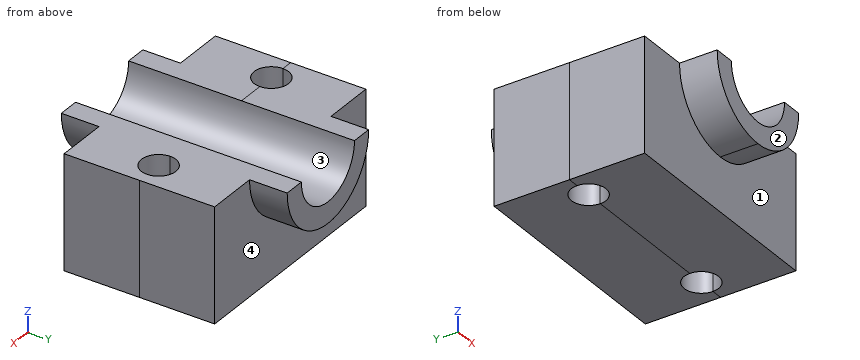
from build123d import *
from build123d import SkipClean  # not in build123d's __all__

# Parameters (mm, degrees)
F1_DEPTH = 25.4
F2_DEPTH = 12.7
F4_DEPTH = 254


with BuildPart() as f1:
    # F0 (on Front) → F1 (new body)
    with BuildSketch(Plane.XZ):
        with BuildLine():
            Line((-37.8727540374, 38.4819693863), (-37.8727540374, 0))
            Line((-37.8727540374, 0), (0, 0))
            Line((0, 0), (0, 18.0733259767))
            ThreePointArc((0, 18.0733259767), (-14.4310901498, 24.0508792366), (-20.4086434096, 38.4819693863))
            Line((-20.4086434096, 38.4819693863), (-37.8727540374, 38.4819693863))
        make_face()
        with BuildLine():
            Line((-13.3011555299, 38.4819693863), (-20.4086434096, 38.4819693863))
            ThreePointArc((-20.4086434096, 38.4819693863), (-14.4310901498, 24.0508792366), (0, 18.0733259767))
            Line((0, 18.0733259767), (0, 25.1808138564))
            ThreePointArc((0, 25.1808138564), (-9.4053372728, 29.0766321135), (-13.3011555299, 38.4819693863))
        make_face()
    extrude(amount=-F1_DEPTH)

    # F0 (on Front) → F2 (join)
    with BuildSketch(Plane.XZ):
        with BuildLine():
            Line((-13.3011555299, 38.4819693863), (-20.4086434096, 38.4819693863))
            ThreePointArc((-20.4086434096, 38.4819693863), (-14.4310901498, 24.0508792366), (0, 18.0733259767))
            Line((0, 18.0733259767), (0, 25.1808138564))
            ThreePointArc((0, 25.1808138564), (-9.4053372728, 29.0766321135), (-13.3011555299, 38.4819693863))
        make_face()
    extrude(amount=F2_DEPTH)

    # F3 (on face) → F4 (cut)
    with BuildSketch(Plane.XY.offset(38.4819693863)):
        with BuildLine():
            ThreePointArc((-34.0433958918, 25.4), (-28.239807114, 19.5964112222), (-22.4362183362, 25.4))
            Line((-22.4362183362, 25.4), (-34.0433958918, 25.4))
        make_face()
    extrude(amount=-F4_DEPTH, mode=Mode.SUBTRACT)

    # F5: F1 across face


with BuildPart() as f1_1:
    add(f1.part, clean=False)
    add(f1.part.mirror(Plane(origin=(0, 10.3439929045, 13.7080154385), x_dir=(0, 1, 0), z_dir=(1, 0, 0))), clean=False)

    # F6: F1 across face


with BuildPart() as f1_2:
    add(f1_1.part, clean=False)
    with SkipClean():  # cleaning this boolean's faces spoils the solid; the shape is the same uncleaned
        add(f1_1.part.mirror(Plane(origin=(0, 25.4, 16.6331926938), x_dir=(-1, 0, 0), z_dir=(0, 1, 0))), clean=False)


solid = f1_2.part
Read the model definition and answer for the solid it produces. Units are mm, in the model's axes. Face numbers are marked on the shaded views. A direction names the side the tool comes from. Round coordinates to 2 decimals unless told otherwise and drop trailing zeros. Order: outer loops, then holes, each group sorted by start corner. A loop starts at its lowest first (then second) coordinate and runs counter-clockwise, first axis right, second up. Notation, with made-up numbers: (3, 85) - (44, 85) arc R24 ccw to (44, 114) - close; hole circle Ø10 at (-9, 79.25). An arc over 180 degrees is marked (long way). Use one line per item in the form item = value. Start each with the question number.
(1) The part is cut by section C-C (y = 23). Give the vertices of the cut face in (x, z), then the cut area to 3 significant figures.
(2) Determine the mould class of the marked faces 3 and 4 for opening direction X: +X half, -X half, draft (parallel to the pull), parting line (faces both ways), or undercut.
(3) The part is cut by section D-D (z = 31.5). Give the vertices of the cut face in (x, y), then the cut area to 3 significant figures.
(4) For the marked faces 1 and 2, determine the directions among +Z, -Z, +X, -X, +Y, -Y from which every point of the face is accessible in a straight line to the end or side of a thin tool.
(5) The part is cut by section A-A (z = 13). Give the vertices of the cut face in (x, y).
(6) The part is cut by section B-B (x = 27). Give the vertices of the cut face in (y, z), then the cut area to 3 significant figures.
(7) Find the intervals of material crossed by line 1 along Y through (x, z) = (28.5, 35); line 2 along X through (y, z) = (21.5, 23); line 3 along X through (y, z) = (29, 19), in increasing order. Write a range as from..to.
Checked values:
q1.outline = (-37.87, 0) - (-33.52, 0) - (-33.52, 38.48) - (-37.87, 38.48) - close; (-22.96, 0) - (22.96, 0) - (22.96, 38.48) - (13.3, 38.48) arc R13.3 cw to (-13.3, 38.48) - (-22.96, 38.48) - close; (33.52, 0) - (37.87, 0) - (37.87, 38.48) - (33.52, 38.48) - close
q1.area = 1,820 mm^2
q2.face_3 = undercut
q2.face_4 = draft
q3.outline = (-37.87, 0) - (-19.18, 0) - (-19.18, -12.7) - (-11.32, -12.7) - (-11.32, 63.5) - (-19.18, 63.5) - (-19.18, 50.8) - (-37.87, 50.8) - close; (11.32, -12.7) - (19.18, -12.7) - (19.18, 0) - (37.87, 0) - (37.87, 50.8) - (19.18, 50.8) - (19.18, 63.5) - (11.32, 63.5) - close; hole circle Ø11.61 at (-28.24, 25.4); hole circle Ø11.61 at (28.24, 25.4)
q3.area = 2,890 mm^2
q4.face_1 = -Z, -Y
q4.face_2 = +Z, -Z, +X, -X, -Y
q5.outline = (-37.87, 0) - (37.87, 0) - (37.87, 50.8) - (-37.87, 50.8) - close; hole circle Ø11.61 at (-28.24, 25.4); hole circle Ø11.61 at (28.24, 25.4)
q6.outline = (0, 0) - (19.73, 0) - (19.73, 38.48) - (0, 38.48) - close; (31.07, 0) - (50.8, 0) - (50.8, 38.48) - (31.07, 38.48) - close
q6.area = 1,520 mm^2
q7.line_1 = 0..19.6, 31.2..50.8
q7.line_2 = -37.87..-32.54, -23.94..23.94, 32.54..37.87
q7.line_3 = -37.87..-32.79, -23.69..23.69, 32.79..37.87
